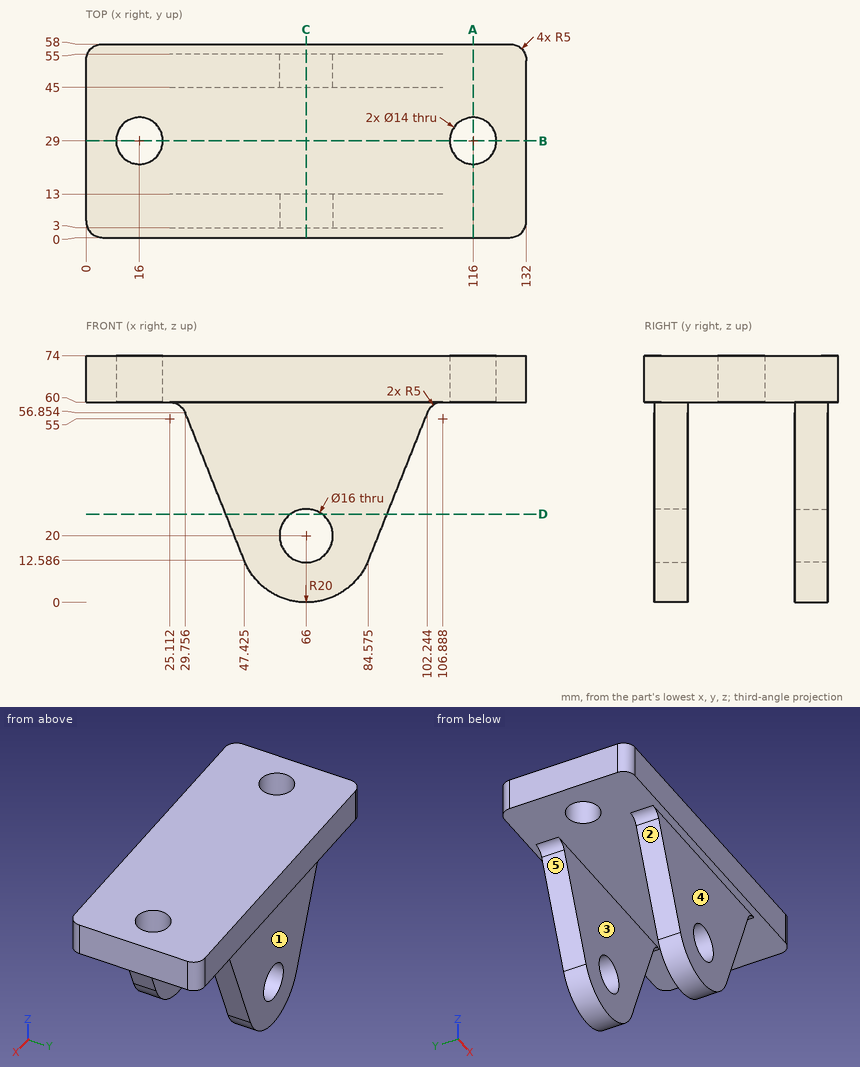
Part print with two shaded views. Sizes in mm from the minimum x, y, z corner. A direction names the side the tool comes from. Give positions to 0.01 mm unless a question says otherwise; leave off trailing zeros. Order: outer loops, then holes, each group sorted by start corner. A loop starts at its lowest first (then second) coordinate and runs counter-clockwise, first axis right, second up.
1) 3-axis set-ups, long thin cutter, end or side, ignore diameter. For the marked faces 1 and 2: which of +Z, -Z, +X, -X, +Y, -Y reach the whole face in a straight line?
2) Pin check, flat tips, straight feed: pin 1 (18 mm diameter, centred on x = 85.5, z = 40.5, fed in from -Y); pin 2 (18 mm diameter, centred on x = 57.5, z = 15.5, fed in from +Y); pin 3 (1 mm diameter, centred on x = 116, y = 21, fed in from -Z); pin 4 (1.5 mm diameter, centred on x = 89.5, z = 63, fed in from -Y). Stop position of each tip, or through.
3) Saw through at C-C, the plane x = 66. Write the cut outline in (y, z).
4) Wall check: probe 1 along Y at (x, z) = (16, 63.5); probe 2 along Y at (x, z) = (66.5, 38); probe 3 along Z at (x, y) = (61, 17). Give the ranges that are in metal, low to high.
5) Saw through at D-D, the plane z = 26.5. Write the cut outline in (x, y).
6) Saw through at B-B, the plane y = 29. Write the cut outline in (x, z), then the cut area to 3 significant figures.
7) Saw through at A-A, the plane x = 116. Write the cut outline in (y, z), then the cut area to 3 significant figures.
8) Mould opens along Y. For the marked faces 3, 4 and 5 say: +Y half, -Y half, draft (parallel to the pull), parting line (faces both ways), or undercut.
Computed:
1. face 1: -Z, +X, -X, +Y
1. face 2: -Z, -X, +Y, -Y
2. pin 1: stops at y = 3
2. pin 2: stops at y = 55
2. pin 3: stops at z = 60
2. pin 4: stops at y = 0
3. outline: (0, 60) - (3, 60) - (3, 28) - (13, 28) - (13, 60) - (45, 60) - (45, 28) - (55, 28) - (55, 60) - (58, 60) - (58, 74) - (0, 74) - close; (3, 0) - (13, 0) - (13, 12) - (3, 12) - close; (45, 0) - (55, 0) - (55, 12) - (45, 12) - close
4. probe 1: y = 0 to 22, 36 to 58
4. probe 2: y = 3 to 13, 45 to 55
4. probe 3: z = 60 to 74
5. outline: (41.87, 3) - (61.34, 3) - (61.34, 13) - (41.87, 13) - close; (41.87, 45) - (61.34, 45) - (61.34, 55) - (41.87, 55) - close; (70.66, 3) - (90.13, 3) - (90.13, 13) - (70.66, 13) - close; (70.66, 45) - (90.13, 45) - (90.13, 55) - (70.66, 55) - close
6. outline: (0, 60) - (9, 60) - (9, 74) - (0, 74) - close; (23, 60) - (109, 60) - (109, 74) - (23, 74) - close; (123, 60) - (132, 60) - (132, 74) - (123, 74) - close
6. area: 1,460 mm2
7. outline: (0, 60) - (22, 60) - (22, 74) - (0, 74) - close; (36, 60) - (58, 60) - (58, 74) - (36, 74) - close
7. area: 616 mm2
8. face 3: undercut
8. face 4: -Y half
8. face 5: draft
